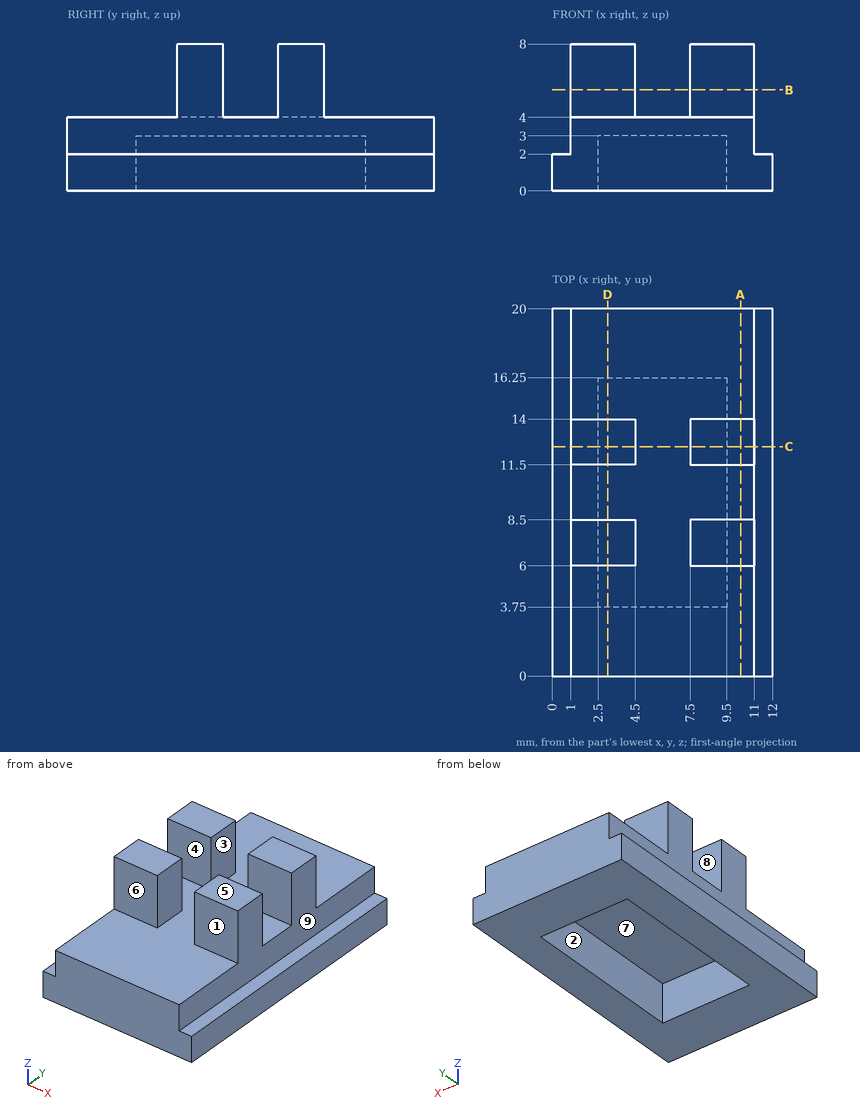
Drawing for the job (mm, zero at the part's lowest x, y, z). A direction names the side the tool comes from. Give positions to 0.01 mm unless a question says otherwise; leave off trailing zeros. Write each loop counter-clockwise with the first axis right and the second up, starting at its lowest first coordinate (ties: lowest second). Pieces come first, ordered by that corner, then holes. Notation, with made-up numbers: (57.25, 29.5) -> (83.25, 29.5) arc R21 ccw to (83.25, 59.5) -> close; hole circle Ø6 at (-25.75, 21.5). An arc over 180 degrees is marked (long way). Put each result on its own line as item: value. Start each with the question number.
Item 1: Pin check, flat tips, straight feed: pin 1 Ø3 at (x, y) = (2.5, 2) entering from +Z; pin 2 Ø1.8 at (y, z) = (7.5, 3.5) entering from -X; pin 3 Ø1 at (y, z) = (3, 6) entering from +X; pin 4 Ø0.5 at (x, y) = (0.5, 15) entering from +Z. Stop position of each tip, or through.
Item 2: Cut at C-C (y = 12.5). List the corners of the cut face in (x, z).
Item 3: Which spindle directions (+Z, -Z, +X, -X, +Y, -Y) get a long thin tool onto all of the face, cutting with end or side? Do the marked faces 1, 2, 3, 4 and 5. Say none if no direction does.
Item 4: Cut at D-D (x = 3). List the corners of the cut face in (y, z), then the cut area to 3 significant figures.
Item 5: Cut at A-A (x = 10.25). List the corners of the cut face in (y, z).
Item 6: Pull direction Y, two halves, no side cores. Call the marked faces 6, 7, 8 and 9: pulls with the +Y half, pulls with the -Y half, needs draft (parallel to the pull), parting line crosses it, or undercut.
Item 7: Wall check: L1, parallel to Y at x = 3.75, z = 5.25; L2, parallel to X at y = 6.5, z = 2.25; L3, parallel to X at y = 7.5, z = 1.5. Give the ranges that are in metal, low to high. Write a range as [from, to].
Item 8: Cut at B-B (z = 5.5). List the corners of the cut face in (x, y).
Answer list:
1. pin 1: stops at z = 4
1. pin 2: stops at x = 1
1. pin 3: passes through
1. pin 4: stops at z = 2
2. outline: (0, 0) -> (2.5, 0) -> (2.5, 3) -> (9.5, 3) -> (9.5, 0) -> (12, 0) -> (12, 2) -> (11, 2) -> (11, 8) -> (7.5, 8) -> (7.5, 4) -> (4.5, 4) -> (4.5, 8) -> (1, 8) -> (1, 2) -> (0, 2) -> close
3. face 1: +Z, +X, -X, -Y
3. face 2: -Z
3. face 3: +Z, +Y, -Y
3. face 4: +Z, +X, -X
3. face 5: +Z, +X, -X, +Y, -Y
4. outline: (0, 0) -> (3.75, 0) -> (3.75, 3) -> (16.25, 3) -> (16.25, 0) -> (20, 0) -> (20, 4) -> (14, 4) -> (14, 8) -> (11.5, 8) -> (11.5, 4) -> (8.5, 4) -> (8.5, 8) -> (6, 8) -> (6, 4) -> (0, 4) -> close
4. area: 62.5 mm2
5. outline: (0, 0) -> (20, 0) -> (20, 4) -> (14, 4) -> (14, 8) -> (11.5, 8) -> (11.5, 4) -> (8.5, 4) -> (8.5, 8) -> (6, 8) -> (6, 4) -> (0, 4) -> close
6. face 6: pulls with the -Y half
6. face 7: undercut
6. face 8: undercut
6. face 9: needs draft
7. L1: y = [6, 8.5], [11.5, 14]
7. L2: x = [1, 2.5], [9.5, 11]
7. L3: x = [0, 2.5], [9.5, 12]
8. outline: (1, 6) -> (4.5, 6) -> (4.5, 8.5) -> (1, 8.5) -> close; (1, 11.5) -> (4.5, 11.5) -> (4.5, 14) -> (1, 14) -> close; (7.5, 6) -> (11, 6) -> (11, 8.5) -> (7.5, 8.5) -> close; (7.5, 11.5) -> (11, 11.5) -> (11, 14) -> (7.5, 14) -> close
